from build123d import *

# Parameters (mm, degrees)
F0_R     = 11.375
F1_DEPTH = 7


with BuildPart() as f1:
    # F0 (on Top) → F1 (new body)
    with BuildSketch(Plane.XY):
        Polygon((-5.591883, -19.115768), (-5.591883, -13.5), (-13.5, -5.591883), (-19.115768, -5.591883), align=None)
        Polygon((-13.5, 5.591883), (-5.591883, 13.5), (-5.591883, 19.115768), (-19.115768, 5.591883), align=None)
        with BuildLine():
            Line((-5.591883, 13.5), (5.591883, 13.5))
            Line((5.591883, 13.5), (5.591883, 19.115768))
            ThreePointArc((5.591883, 19.115768), (8.736079, 29.565264), (0, 36.104289))
            ThreePointArc((0, 36.104289), (-8.736079, 29.565264), (-5.591883, 19.115768))
            Line((-5.591883, 19.115768), (-5.591883, 13.5))
        make_face()
        Polygon((2.744165, 33.255364), (6.625, 29.374529), (6.625, 23.8862), (2.744165, 20.005364), (-2.744165, 20.005364), (-6.625, 23.8862), (-6.625, 29.374529), (-2.744165, 33.255364), align=None, mode=Mode.SUBTRACT)
        with BuildLine():
            Line((-13.5, -5.591883), (-13.5, 5.591883))
            Line((-13.5, 5.591883), (-19.115768, 5.591883))
            ThreePointArc((-19.115768, 5.591883), (-29.565264, 8.736079), (-36.104289, 0))
            ThreePointArc((-36.104289, 0), (-29.565264, -8.736079), (-19.115768, -5.591883))
            Line((-19.115768, -5.591883), (-13.5, -5.591883))
        make_face()
        Polygon((-20.005364, 2.744165), (-20.005364, -2.744165), (-23.8862, -6.625), (-29.374529, -6.625), (-33.255364, -2.744165), (-33.255364, 2.744165), (-29.374529, 6.625), (-23.8862, 6.625), align=None, mode=Mode.SUBTRACT)
        Polygon((5.591883, 13.5), (13.5, 5.591883), (19.115768, 5.591883), (5.591883, 19.115768), align=None)
        with BuildLine():
            Line((19.115768, 5.591883), (13.5, 5.591883))
            Line((13.5, 5.591883), (13.5, -5.591883))
            Line((13.5, -5.591883), (19.115768, -5.591883))
            ThreePointArc((19.115768, -5.591883), (29.565264, -8.736079), (36.104289, 0))
            ThreePointArc((36.104289, 0), (29.565264, 8.736079), (19.115768, 5.591883))
        make_face()
        Polygon((20.005364, -2.744165), (20.005364, 2.744165), (23.8862, 6.625), (29.374529, 6.625), (33.255364, 2.744165), (33.255364, -2.744165), (29.374529, -6.625), (23.8862, -6.625), align=None, mode=Mode.SUBTRACT)
        Polygon((19.115768, -5.591883), (13.5, -5.591883), (5.591883, -13.5), (5.591883, -19.115768), align=None)
        with BuildLine():
            Line((5.591883, -19.115768), (5.591883, -13.5))
            Line((5.591883, -13.5), (-5.591883, -13.5))
            Line((-5.591883, -13.5), (-5.591883, -19.115768))
            ThreePointArc((-5.591883, -19.115768), (-8.736079, -29.565264), (0, -36.104289))
            ThreePointArc((0, -36.104289), (8.736079, -29.565264), (5.591883, -19.115768))
        make_face()
        Polygon((-2.744165, -20.005364), (2.744165, -20.005364), (6.625, -23.8862), (6.625, -29.374529), (2.744165, -33.255364), (-2.744165, -33.255364), (-6.625, -29.374529), (-6.625, -23.8862), align=None, mode=Mode.SUBTRACT)
        Polygon((13.5, -5.591883), (13.5, 5.591883), (5.591883, 13.5), (-5.591883, 13.5), (-13.5, 5.591883), (-13.5, -5.591883), (-5.591883, -13.5), (5.591883, -13.5), align=None)
        Circle(F0_R, mode=Mode.SUBTRACT)
    extrude(amount=F1_DEPTH)


solid = f1.part
Check sheet for the modelled part. Datum: model origin and axes. Units: mm. A direction names the side the tool comes from. Round coordinates to 2 decimals unless told otherwise and drop trailing zeros. Loops run counter-clockwise (first coordinate to the right, second up) from the corner with the lowest first, then second, coordinate; pieces in that order, holes last. Notation, with made-up numbers: (71, -35) - (121, -35) arc R21 ccw to (121, -5) - close; hole circle Ø7 at (23, -26.75). An arc over 180 degrees is marked (long way). Answer as CSV lines item,"result". Start each with the question number.
Item 1: Depth check by flat-ended pin: P1, Ø2.5, axis at y = -27.5, z = 4, coming from the -X side; P2, Ø2.5, axis at x = -27.5, z = 2.5, coming from the -Y side; P3, Ø1.5, axis at x = 10.5, z = 3.5, coming from the -Y side. Enter the tip coordinate at first touch or a pass-through.
Item 2: Section check B-B (x = 1). Record the boundary of the cut face in (y, z), and give its area (3 significant figures).
Item 3: Release check for a two-part mould opening along Y. For faces 1 (the flat face through (-27, -6.625, 3)), 2 (the flat face through (5, -11, 7)) record: +Y half, -Y half, draft (parallel to the pull), parting line (faces both ways), or undercut.
Item 4: Set-up check for faces 3 (the cylindrical face through (-8.786, -29.41, 3.451)), 4 (the flat face through (4.66, -21.92, 3.45)): record each of +Z, -Z, +X, -X, +Y, -Y from which the full face is reachable in a straight line by a thin tool's end or side.
Item 5: Section check C-C (z = 4). Count the separate pieces of the cut face and the enclosed holes in it, and give its area (3 significant figures).
Item 6: Scan lines: line 1 (Y direction, x = 8, z = 5.5); line 2 (X direction, y = -3, z = 5.25); line 3 (Y direction, x = -7, z = 3). Record each from-to range of solid material in increasing order. Write a range as [from, to].
Item 7: Section check A-A (y = 26). Record the boundary of the cut face in (x, z) (3 decimals).
Item 8: Section check D-D (y = -14). Record the boundary of the cut face in (x, z).
Report:
1,P1,"stops at x = -9.21"
1,P2,"stops at y = -9.21"
1,P3,"stops at y = -14.96"
2,outline,"(-36.02, 0) - (-33.26, 0) - (-33.26, 7) - (-36.02, 7) - close; (-20.01, 0) - (-11.33, 0) - (-11.33, 7) - (-20.01, 7) - close; (11.33, 0) - (20.01, 0) - (20.01, 7) - (11.33, 7) - close; (33.26, 0) - (36.02, 0) - (36.02, 7) - (33.26, 7) - close"
2,area,"160 mm2"
3,face 1,"undercut"
3,face 2,"draft"
4,face 3,"+Z, -Z, -X"
4,face 4,"+Z, -Z"
5,separate pieces,"1"
5,enclosed holes,"5"
5,area,"1,140 mm2"
6,line 1,"y = [-31.24, -21.94], [-16.71, -8.09], [8.09, 16.71], [21.94, 31.24]"
6,line 2,"x = [-35.52, -33], [-20.26, -10.97], [10.97, 20.26], [33, 35.52]"
6,line 3,"y = [-32.69, -20.49], [-17.71, -8.97], [8.97, 17.71], [20.49, 32.69]"
7,outline,"(-9.195, 0) - (-6.625, 0) - (-6.625, 7) - (-9.195, 7) - close; (6.625, 0) - (9.195, 0) - (9.195, 7) - (6.625, 7) - close"
8,outline,"(-10.71, 0) - (10.71, 0) - (10.71, 7) - (-10.71, 7) - close"
